from build123d import *

# Parameters (mm, degrees)
SKETCH1_R               = 1.5
BOSS_EXTRUDE1_DEPTH     = 10
SKETCH2_R               = 2
CUT_EXTRUDE1_DEPTH      = 30
SKETCH6_R               = 7.5
BOSS_EXTRUDE3_DEPTH     = 5
CUT_EXTRUDE4_DEPTH      = 26.013853674
CUT_EXTRUDE4_DEPTH_BACK = 26.013853674
SKETCH7_R               = 1.5
SKETCH8_R               = 2
CUT_EXTRUDE5_DEPTH      = 18
SKETCH10_R              = 7.5
CUT_EXTRUDE7_DEPTH      = 9
SKETCH11_W              = 8
SKETCH11_H              = 8
BOSS_EXTRUDE4_DEPTH     = 5
SKETCH13_R              = 1.5
CUT_EXTRUDE8_DEPTH      = 10


with BuildPart() as part:
    # Sketch1 → Boss-Extrude1 (new body)
    with BuildSketch(Plane.XY):
        with BuildLine():
            Line((5.026455026, -10.023549892), (-4.973544974, -10.023549892))
            Line((-4.973544974, -10.023549892), (-4.973544974, 4.386280164))
            ThreePointArc((-4.973544974, 4.386280164), (0.026455026, 17.476450108), (5.026455026, 4.386280164))
            Line((5.026455026, 4.386280164), (5.026455026, -10.023549892))
        make_face()
        with Locations((0.026455026, 9.976450108)):
            Circle(SKETCH1_R, mode=Mode.SUBTRACT)
    extrude(amount=BOSS_EXTRUDE1_DEPTH)

    # Sketch2 → Cut-Extrude1 (cut)
    with BuildSketch(Plane(origin=(0, 0, 0), x_dir=(-1, 0, 0), z_dir=(0, 0, -1))):
        with Locations((-0.026455026, 9.976450108)):
            Circle(SKETCH2_R)
    extrude(amount=-CUT_EXTRUDE1_DEPTH, mode=Mode.SUBTRACT)

    # Sketch6 → Boss-Extrude3 (add, symmetric)
    with BuildSketch(Plane(origin=(2.513227513, 0, 2.513227513), x_dir=(-0.7071067811865477, 0, 0.7071067811865475), z_dir=(-0.7071067811865475, 0, -0.7071067811865477))):
        with Locations((3.516827377, -10.023549892)):
            Circle(SKETCH6_R)
    extrude(amount=BOSS_EXTRUDE3_DEPTH, both=True)

    # Sketch7 → Cut-Extrude4 (cut, two sides: drawn at the far end of the back side and taken through both)
    with BuildSketch(Plane(origin=(-1.022306393, 0, -1.022306393), x_dir=(-0.7071067811865476, 0, 0.7071067811865476), z_dir=(-0.7071067811865476, 0, -0.7071067811865476)).offset(-CUT_EXTRUDE4_DEPTH_BACK)):
        with Locations((3.516827377, -10.023549892)):
            Circle(SKETCH7_R)
    extrude(amount=CUT_EXTRUDE4_DEPTH + CUT_EXTRUDE4_DEPTH_BACK, mode=Mode.SUBTRACT)

    # Sketch8 → Cut-Extrude5 (cut, symmetric)
    with BuildSketch(Plane(origin=(-1.022306393, 0, -1.022306393), x_dir=(-0.7071067811865476, 0, 0.7071067811865476), z_dir=(-0.7071067811865476, 0, -0.7071067811865476))):
        with Locations((3.516827377, -10.023549892)):
            Circle(SKETCH8_R)
    extrude(amount=CUT_EXTRUDE5_DEPTH, both=True, mode=Mode.SUBTRACT)

    # Sketch10 → Cut-Extrude7 (cut)
    with BuildSketch(Plane(origin=(6.048761419, 0, 6.048761419), x_dir=(0.7071067811865476, 0, -0.7071067811865476), z_dir=(0.7071067811865476, 0, 0.7071067811865476))):
        with Locations((-3.516827377, -10.023549892)):
            Circle(SKETCH10_R)
    cut_extrude7 = extrude(amount=CUT_EXTRUDE7_DEPTH, mode=Mode.SUBTRACT)

    # Mirror1: Cut-Extrude7 across plane
    add(cut_extrude7.mirror(Plane(origin=(2.513227513, 0, 2.513227513), x_dir=(-0.7071067811865478, 0, 0.7071067811865472), z_dir=(-0.7071067811865475, 0, -0.7071067811865477))), mode=Mode.SUBTRACT)

    # Sketch11 → Boss-Extrude4 (add, symmetric)
    with BuildSketch(Plane(origin=(0, -17.5, 0), x_dir=(1, 0, 0), z_dir=(0, 1, 0))):
        with Locations((-0.219742317, -5.27916127)):
            Rectangle(SKETCH11_W, SKETCH11_H)
    extrude(amount=BOSS_EXTRUDE4_DEPTH, both=True)

    # Sketch13 → Cut-Extrude8 (cut)
    with BuildSketch(Plane(origin=(3.780257683, 0, 0), x_dir=(0, 0, -1), z_dir=(1, 0, 0))):
        with Locations((-5, -19.771629817)):
            Circle(SKETCH13_R)
        Polygon((-5.836861044, -21.653637688), (-9.27916127, -17.5), (-9.27916127, -22.5), (-1.27916127, -22.5), (-1.27916127, -17.51897011), (-3.745741187, -21.653637688), align=None)
    extrude(amount=-CUT_EXTRUDE8_DEPTH, mode=Mode.SUBTRACT)


solid = part.part
Part model, mm, in its own coordinate system. A direction names the side the tool comes from. Coordinates: 2 decimals unless noted, no trailing zeros. Loops run counter-clockwise (first coordinate to the right, second up) from the corner with the lowest first, then second, coordinate; pieces in that order, holes last. Notation, with made-up numbers: M 8.25,19 L 24.25,19 A23 ccw 24.25,38 Z; hole C -5.75,-35.5 d4. An arc over 180 degrees is marked long. Use a Markdown table: item, result. Add a question column.
Q1. Probe L1, parallel to Y at x = 0.5, z = 5; L2, parallel to Y at x = -1.5, z = 5; L3, parallel to X at y = -18, z = 6.5. List the from-to ranges inside material, lowest first.
Q2. Cut at A-A (y = -8.5). Write the cut outline in (x, z).
Q3. Cut at D-D (y = 9.5). Write the cut outline in (x, z), and give its area (3 significant figures).
Q4. Mould opens along X. For faces 5 (the cylindrical face through (0.16, -8.04, 4.77)), 6 (the flat face through (-4.974, 0, 5)), 7 (the cylindrical face through (-0.164, -18.284, 5.195)) say: +X half, -X half, draft (parallel to the pull), parting line (faces both ways), or undercut.
Q5. Which spindle directions (+Z, -Z, +X, -X, +Y, -Y) get a long thin tool onto all of the face, cutting with end or side? Do faces 1 (the flat face through (-4, -15, 1.279)), 2 (the flat face through (-4.22, -18, 5)), 3 (the flat face through (3.78, -18, 6)), 4 (the flat face through (-1, -17, 9.279)). Say none if no direction does.
Q6. Cut at B-B (z = 4.5). Give the number of separate pieces and of enclosed holes in the cut face, and give its area (3 significant figures).
Q7. Cut at C-C (y = -2). Write the cut outline in (x, z).
Q8. Pin check, flat tips, straight feed: P1, Ø5, axis at y = -19.77, z = 5, coming from the -X side; P2, Ø4, axis at y = 6.5, z = 7, coming from the -X side; P3, Ø5, axis at y = 7.5, z = 0.5, coming from the -X side. Stop position of each tip, or through.
Worked out:
| question | item | result |
|---|---|---|
| 1 | L1 | y = -21.65 to -21.27, -18.27 to -12, -8.05 to 8.03, 11.92 to 17.46 |
| 1 | L2 | y = -21.65 to -21.27, -18.27 to -11.71, -8.34 to 8.68, 11.27 to 17.32 |
| 1 | L3 | x = -4.22 to 3.78 |
| 2 | outline | M -8.7,6.66 L -4.43,2.38 L 2.65,9.45 L -1.63,13.73 Z; M -2.59,0.55 L 1.68,-3.73 L 8.75,3.34 L 4.48,7.62 Z |
| 3 | outline | M -7.46,0 L -1.92,0 L -1.92,10 L -7.46,10 Z; M 1.97,0 L 7.51,0 L 7.51,10 L 1.97,10 Z |
| 3 | area | 111 mm2 |
| 4 | face 5 | undercut |
| 4 | face 6 | -X half |
| 4 | face 7 | draft |
| 5 | face 1 | -Z, -X, -Y |
| 5 | face 2 | -X, -Y |
| 5 | face 3 | +X, -Y |
| 5 | face 4 | +Z, -Y |
| 6 | separate pieces | 2 |
| 6 | enclosed holes | 2 |
| 6 | area | 411 mm2 |
| 7 | outline | M -4.97,0 L 5.03,0 L 5.03,10 L -4.97,10 Z |
| 8 | P1 | stops at x = -4.22 |
| 8 | P2 | stops at x = -7.33 |
| 8 | P3 | stops at x = -7.47 |
